Geometry: final body of the model. Coordinates: model frame, mm. A direction names the side the tool comes from. Round coordinates to 2 decimals unless told otherwise and drop trailing zeros. Order: outer loops, then holes, each group sorted by start corner. A loop starts at its lowest first (then second) coordinate and runs counter-clockwise, first axis right, second up. Notation, with made-up numbers: (32, 12) -> (48, 12) arc R32 cw to (48, 40) -> close; hole circle Ø8 at (33, 83.5). An arc over 180 degrees is marked (long way). Put each result on its own line as item: value.
```python
from build123d import *

# Parameters (mm, degrees)
F0_W     = 80
F0_H     = 50
F1_DEPTH = 50
F4_DEPTH = 10
F5_W     = 15
F5_H     = 10
F6_DEPTH = 25
F7_DEPTH = 10
F9_DEPTH = 10


with BuildPart() as f1:
    # F0 (on Front) → F1 (new body)
    with BuildSketch(Plane.XZ):
        with Locations((40, 25)):
            Rectangle(F0_W, F0_H)
    extrude(amount=F1_DEPTH)

    # F2 (on face) → F4 (cut)
    with BuildSketch(Plane.XY.offset(50)):
        Polygon((70, 0), (40, 0), (50, -50), (60, -50), align=None)
    extrude(amount=-F4_DEPTH, mode=Mode.SUBTRACT)

    # F5 (on face) → F6 (cut)
    with BuildSketch(Plane.YZ.offset(80)):
        with Locations((-36.5, 30)):
            Rectangle(F5_W, F5_H)
        Polygon((-29, 35), (-29, 25), (-24, 25), align=None)
    extrude(amount=-F6_DEPTH, mode=Mode.SUBTRACT)

    # F5 (on face) → F7 (cut)
    with BuildSketch(Plane.YZ.offset(80)):
        Polygon((0, 10), (-12, 0), (0, 0), align=None)
    extrude(amount=-F7_DEPTH, mode=Mode.SUBTRACT)

    # F8 (on face) → F9 (cut)
    with BuildSketch(Plane(origin=(0, 0, 0), x_dir=(1, 0, 0), z_dir=(0, 0, -1))):
        Polygon((20, 50), (30, 0), (40, 0), (50, 50), align=None)
    extrude(amount=-F9_DEPTH, mode=Mode.SUBTRACT)

    # F12: sweep along a path in F3
    with BuildLine(Plane(origin=(0, 0, 0), x_dir=(0, -1, 0), z_dir=(-1, 0, 0))) as f12_path:
        Line((50, 15), (0, 25))
    # F11 (on face) → F12 (sweep, cut)
    with BuildSketch(Plane.XZ.offset(50)):
        Polygon((0, 15), (30, 50), (0, 50), align=None)
    sweep(path=f12_path.line, mode=Mode.SUBTRACT)


solid = f1.part
```
1. Set-up query: faces 4 (the face through (70, -3, 3)), 5 (the face through (68, -37, 35)), 6 (the face through (45, -25, 45)). Return all of +Z, -Z, +X, -X, +Y, -Y with unobstructed straight access to the full face (end or side cutting, diameter ignored); none if empty.
Ans:
face 4: -Z, +X, +Y
face 5: +X
face 6: +Z, +Y
2. Contact query for flat-ended pins moving along their axis: P1, Ø6, axis at y = -13.5, z = 35, coming from the -X side; P2, Ø4, axis at x = 9, z = 41.5, coming from the +Y side; P3, Ø3, axis at y = -31, z = 30, coming from the +X side; P4, Ø6, axis at x = 20.5, y = -20, coming from the +Z side. Output: stop coordinate, or through.
Ans:
P1: x = 8.26
P2: through
P3: x = 55
P4: z = 48.47
3. Material intervals for probe 1 along Z at (x, y) = (31, -39); probe 2 along X at (y, z) = (-39, 5); probe 3 along X at (y, z) = (-21, 7), sorted ascending.
Ans:
probe 1: 10 to 50
probe 2: 0 to 22.2, 47.8 to 80
probe 3: 0 to 25.8, 44.2 to 80
4. Draft query along Z for faces 1 (the face through (65, -25, 45)), 2 (the face through (35, -31, 10)), 3 (the face through (68, -34, 25)). Return one class per face: +Z half, -Z half, draft (parallel to the pull), parting line (faces both ways), or undercut.
Ans:
face 1: draft
face 2: -Z half
face 3: undercut
5. Cut plane C-C on z = 47. Return loops of the section in (x, y).
Ans:
outline: (18.86, 0) -> (27.43, -50) -> (50, -50) -> (40, 0) -> close; (60, -50) -> (80, -50) -> (80, 0) -> (70, 0) -> close
6. Cut plane A-A on x = 63. Return loops of the section in (y, z), and give its area (4 significant figures).
Ans:
outline: (-50, 0) -> (0, 0) -> (0, 40) -> (-35, 40) -> (-35, 50) -> (-50, 50) -> close; hole (-44, 25) -> (-24, 25) -> (-29, 35) -> (-44, 35) -> close
area: 1,975 mm²
7. Cut plane B-B on y = -36. Return loops of the section in (x, z), and give its area (3 significant figures).
Ans:
outline: (0, 0) -> (22.8, 0) -> (22.8, 10) -> (47.2, 10) -> (47.2, 0) -> (80, 0) -> (80, 25) -> (55, 25) -> (55, 35) -> (80, 35) -> (80, 50) -> (62.8, 50) -> (62.8, 40) -> (47.2, 40) -> (47.2, 50) -> (27.6, 50) -> (0, 17.8) -> close
area: 2,910 mm²
8. Cut plane D-D on x = 44. Return loops of the section in (y, z).
Ans:
outline: (-50, 10) -> (-20, 10) -> (-20, 0) -> (0, 0) -> (0, 40) -> (-20, 40) -> (-20, 50) -> (-50, 50) -> close
